Source: CAD feature listing. Evaluate the final solid. Frame: model axes, mm. A direction names the side the tool comes from. Round coordinates to 2 decimals unless told otherwise and drop trailing zeros. Loops run counter-clockwise (first coordinate to the right, second up) from the corner with the lowest first, then second, coordinate; pieces in that order, holes last. Notation, with made-up numbers: (60, 19) - (118, 19) arc R23 ccw to (118, 32) - close; hole circle Ø4 at (-14.5, 59). An arc over 180 degrees is marked (long way). One line per question, with ' | ' between items. Start each with the question number.
1. Cut plane C-C (x = -2.5). Return loops of the section in (y, z).
2. Mould query, pull axis X, two halves, no side actions, for faces 1 (the flat face through (38, 0, -18)), 2 (the cylindrical face through (73, -3, 0)), 3 (the flat face through (99.57, -5.42, -9.21)). Classes: pulls with the +X half, pulls with the -X half, needs draft (parallel to the pull), parting line crosses it, or undercut.
3. Ray query, line 1 (Y direction, x = -11.5, z = 8); line 2 (X direction, y = -17.1, z = 0); line 3 (Z direction, x = 19, y = -12.5). Return the intervals inside material, ascending.
4. Access query for faces 4 (the flat face through (39, -10, -16.5)), 5 (the flat face through (-5, -14, 0)), 6 (the cylindrical face through (73, -17, 0)). Directions: +Z, -Z, +X, -X, +Y, -Y. A direction counts if a zero-diameter tool reaches every point of the face in a straight line with its end or side. Return the directions, or none.
5. Cut plane D-D (z = 10). Return loops of the section in (x, y).
6. Cut plane A-A (y = -4.5). Return loops of the section in (x, z).
7. Pin query (flat end, axial travel): pin 1 (13 mm diameter, centred on x = 77, z = 0, fed in from +Y); pin 2 (10 mm diameter, centred on y = -15, z = -10, fed in from +X); pin 3 (8 mm diameter, centred on y = -11, z = -6, fed in from -X); pin 4 (10 mm diameter, centred on x = 54.5, y = -7, fed in from +Z). Return the tip coordinate at first contact, or that it passes through.
8. Cut plane B-B (z = -1.5). State how many separate pieces and enclosed holes the cut face has, then the cut area to 3 significant figures.
```python
from build123d import *

# Parameters (mm, degrees)
F0_R          = 4
F1_DEPTH      = 20
F2_W          = 8
F2_H          = 60.2939470698
F3_DEPTH      = 128.3
F3_DEPTH_BACK = 41.8


with BuildPart() as f1:
    # F0 (on Front) → F1 (new body)
    with BuildSketch(Plane.XZ):
        with BuildLine():
            Line((77, -16.5), (0, -16.5))
            ThreePointArc((0, -16.5), (13.9314518969, 8.8410773125), (-14.9295810055, 7.0254972066))
            Line((-14.9295810055, 7.0254972066), (-30, -25))
            Line((-30, -25), (107, -25))
            Line((107, -25), (91.9295810055, 7.0254972066))
            ThreePointArc((91.9295810055, 7.0254972066), (63.0685481031, 8.8410773125), (77, -16.5))
        make_face()
        Circle(F0_R, mode=Mode.SUBTRACT)
        with Locations((77, 0)):
            Circle(F0_R, mode=Mode.SUBTRACT)
    extrude(amount=F1_DEPTH)

    # F2 (on Right) → F3 (cut, two sides)
    with BuildSketch(Plane.YZ) as f3_sk:
        with Locations((-10, 13.6469735349)):
            Rectangle(F2_W, F2_H)
    extrude(amount=F3_DEPTH, mode=Mode.SUBTRACT)
    extrude(f3_sk.sketch, amount=-F3_DEPTH_BACK, mode=Mode.SUBTRACT)


solid = f1.part
```
Answers follow:
1) outline: (-20, -25) - (0, -25) - (0, -3.12) - (-6, -3.12) - (-6, -16.5) - (-14, -16.5) - (-14, -3.12) - (-20, -3.12) - close; (-20, 3.12) - (-14, 3.12) - (-14, 16.31) - (-20, 16.31) - close; (-6, 3.12) - (0, 3.12) - (0, 16.31) - (-6, 16.31) - close
2) face 1: needs draft | face 2: undercut | face 3: pulls with the +X half
3) line 1: y = -20 to -14, -6 to 0 | line 2: x = -18.24 to -4, 4 to 16.5, 60.5 to 73, 81 to 95.24 | line 3: z = -25 to -16.5
4) face 4: none | face 5: +Z, +X, -X | face 6: +Y, -Y
5) outline: (-13.12, -20) - (13.12, -20) - (13.12, -14) - (-13.12, -14) - close; (-13.12, -6) - (13.12, -6) - (13.12, 0) - (-13.12, 0) - close; (63.88, -20) - (90.12, -20) - (90.12, -14) - (63.88, -14) - close; (63.88, -6) - (90.12, -6) - (90.12, 0) - (63.88, 0) - close
6) outline: (-30, -25) - (107, -25) - (91.93, 7.03) arc R16.5 ccw (long way) to (77, -16.5) - (0, -16.5) arc R16.5 ccw (long way) to (-14.93, 7.03) - close; hole circle Ø8 at (0, 0); hole circle Ø8 at (77, 0)
7) pin 1: stops at y = 0 | pin 2: stops at x = 102.29 | pin 3: stops at x = -22.3 | pin 4: stops at z = -16.5
8) separate pieces: 8 | enclosed holes: 0 | area: 671 mm2
